Part print with two shaded views. Sizes in mm from the minimum x, y, z corner. A direction names the side the tool comes from. Give positions to 0.01 mm unless a question says otherwise; leave off trailing zeros. Write each loop counter-clockwise with the first axis right and the second up, starting at its lowest first coordinate (ties: lowest second). Pieces come first, ordered by that corner, then holes. Notation, with made-up numbers: (-25, -19) -> (-17, -19) arc R33 cw to (-17, 16) -> close; hole circle Ø5 at (67.5, -28.75). An arc over 180 degrees is marked (long way). Answer as a JSON object with one key per item and string values.
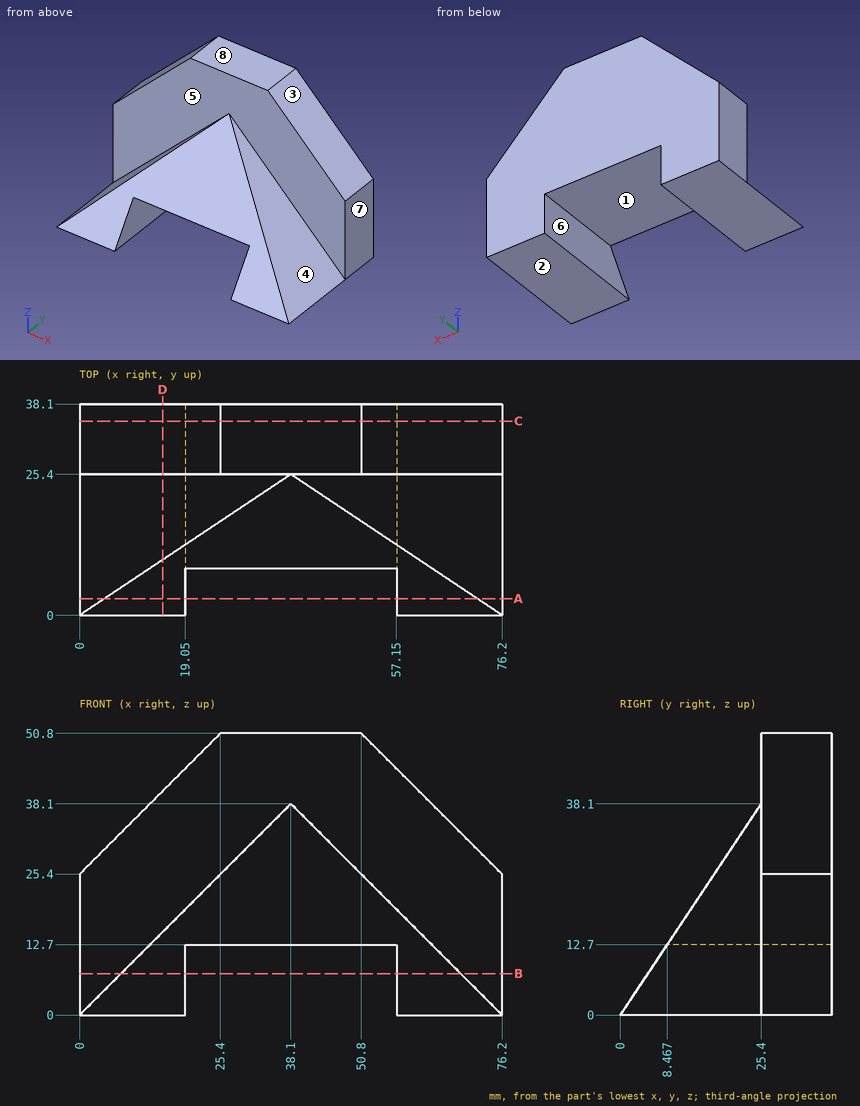
1) Slice it at A-A (y = 3). List the corners of the cut face in (x, z).
Model answer:
{"outline": "(0, 0) -> (19.05, 0) -> (19.05, 4.5) -> (4.5, 4.5) -> close; (57.15, 0) -> (76.2, 0) -> (71.7, 4.5) -> (57.15, 4.5) -> close"}
2) Slice it at C-C (y = 35). List the corners of the cut face in (x, z).
Model answer:
{"outline": "(0, 0) -> (19.05, 0) -> (19.05, 12.7) -> (57.15, 12.7) -> (57.15, 0) -> (76.2, 0) -> (76.2, 25.4) -> (50.8, 50.8) -> (25.4, 50.8) -> (0, 25.4) -> close"}
3) 3-axis set-ups, long thin cutter, end or side, ignore diameter. For the marked faces 1, 2, 3, 4 and 5: which of +Z, -Z, +X, -X, +Y, -Y reach the whole face in a straight line?
Model answer:
{"face 1": "-Z, +Y, -Y", "face 2": "-Z, +X, -X, +Y, -Y", "face 3": "+Z, +X, +Y, -Y", "face 4": "+Z, +X, -Y", "face 5": "+Z, -Y"}
4) Mould opens along X. For the marked faces 6, 7 and 8 say: released by +X, released by -X, zero draft, split by the parting line, or undercut.
Model answer:
{"face 6": "undercut", "face 7": "released by +X", "face 8": "zero draft"}
5) Slice it at D-D (x = 15). List the corners of the cut face in (y, z).
Model answer:
{"outline": "(0, 0) -> (38.1, 0) -> (38.1, 40.4) -> (25.4, 40.4) -> (25.4, 15) -> (10, 15) -> close"}
6) Wall check: probe 1 along X at (y, z) = (4.5, 6); probe 2 along X at (y, z) = (19, 9); probe 3 along Z at (x, y) = (63.5, 19). Give the ranges that are in metal, low to high.
Model answer:
{"probe 1": "x = 6 to 19.05, 57.15 to 70.2", "probe 2": "x = 9 to 19.05, 57.15 to 67.2", "probe 3": "z = 0 to 12.7"}
7) Slice it at B-B (z = 7.5). List the corners of the cut face in (x, y), then the cut area to 3 significant figures.
Model answer:
{"outline": "(0, 25.4) -> (7.5, 25.4) -> (7.5, 5) -> (19.05, 5) -> (19.05, 38.1) -> (0, 38.1) -> close; (57.15, 5) -> (68.7, 5) -> (68.7, 25.4) -> (76.2, 25.4) -> (76.2, 38.1) -> (57.15, 38.1) -> close", "area": "955 mm2"}
8) Pin check, flat tips, straight feed: pin 1 (6 mm diameter, centred on x = 21, z = 16, fed in from -Y); pin 2 (1 mm diameter, centred on x = 54, y = 25.5, fed in from -Z); pin 3 (1 mm diameter, centred on y = 22.5, z = 30, fed in from +X). Stop position of each tip, or through.
Model answer:
{"pin 1": "stops at y = 8.67", "pin 2": "stops at z = 12.7", "pin 3": "stops at x = 46.7"}
